Model file for the job. Use its own axes, mm. A direction names the side the tool comes from. Coordinates: 2 decimals unless noted, no trailing zeros. Write each loop counter-clockwise with the first axis right and the second up, starting at its lowest first coordinate (ties: lowest second). Pieces come first, ordered by that corner, then holes. Notation, with made-up numbers: M -3.75,54 L 49.25,54 A29 cw 49.25,74 Z; hole C 9.25,-6 d1. An arc over 180 degrees is marked long. Use CSV: the item, a comma, the result in double quotes. Start each with the question number.
Autodesk Fusion 360 part; units mm, degrees
sketch "Sketch1" plane through (0, 0, 0) normal (0, 0, 1) x (1, 0, 0)
  line L0 (0, 0) -> (20, 0)
  line L1 (20, 0) -> (20, 11)
  line L2 (20, 11) -> (0, 11)
  line L3 (0, 11) -> (0, 0)
  line L4 (0, 0) -> (80, 0)
  line L5 (0, 11) -> (0, 26)
  line L6 (0, 26) -> (80, 26)
  line L7 (80, 26) -> (80, 0)
  line L8 (80, 0) -> (0, 0)
  line L9 (0, 0) -> (0, 26)
  line L10 (80, 0) -> (80, -10)
  line L11 (80, -10) -> (0, -10)
  line L12 (0, -10) -> (0, 0)
  point P0 (5.75, 9.5)
  point P1 (14.25, 9.5)
  point P2 (14.25, 1.5)
  point P3 (5.75, 1.5)
  dimension "d1" = 20
  dimension "d2" = 11
  dimension "d3" = 1.5
  dimension "d4" = 1.5
  dimension "d5" = 8.5
  dimension "d6" = 5.75
  dimension "d7" = 80
  dimension "d8" = 15
  dimension "d19" = 10
extrude "Extrude1" add sketch "Sketch1" along normal blind 5
hole "Hole1" at (14.25, 1.5, 0) direction (0, 0, 1) diameter 2 end through all
pattern_linear "R-Pattern1" count 2 spacing 8.5 along (-1, 0, 0) count 2 spacing 8 along (0, 1, 0) of "Hole1"
sketch "Sketch2" plane through (0, 26, 0) normal (0, 1, 0) x (-1, 0, 0)
  line L0 (-80, 0) -> (0, 0)
  line L1 (0, 0) -> (0, 5)
  line L2 (0, 5) -> (-80, 5)
  line L3 (-80, 5) -> (-80, 0)
  circle A0 centre (-65, 25) radius 8
  line L4 (-73, 25) -> (-73, 5)
  line L5 (-57, 25) -> (-57, 5)
  line L6 (-57, 5) -> (-73, 5)
  circle A1 centre (-65, 25) radius 10
  line L7 (-75, 25) -> (-75, 5)
  line L8 (-55, 25) -> (-55, 5)
  dimension "d24" = 16
  dimension "d25" = 7
  dimension "d27" = 20
  dimension "d28" = 2
  dimension "d29" = 2
  dimension "d30" = -2
extrude "Extrude2" add sketch "Sketch2" against normal blind 5 contours L2 L4 A1 L7 | L2 L5 A1 L8 | L2 L4 L5 L6 A1 | A0 L4 L5 A1 | A0 L4 L5 A1
ref_plane "WorkPlane2" through (65, 15.5, 20) normal (0, -1, 0) x (1, 0, 0)
mirror "Mirror1" about plane through (65, 15.5, 20) normal (0, -1, 0) of "Extrude2"
equation "d33 = ( 11 / 2 ) * 1 mm"
1) Two-plate mould, pull along X, no slides. Class faces 1 (the face through (80, 8, 2)), 2 (the face through (39, 8, 5)), 3 (the face through (15.226, 1.283, 2.535)): pulls with the +X half, pulls with the -X half, needs draft (parallel to the pull), parting line crosses it, or undercut.
2) Band-saw the part on B-B on z = 12.5. List the corners of the cut face in (x, y).
3) Band-saw the part on D-D on z = 29.5. List the corners of the cut face in (x, y), then the cut area to 3 significant figures.
4) Band-saw the part on C-C on y = 1.5. List the corners of the cut face in (x, z), then the cut area to 3 significant figures.
5) Band-saw the part on A-A on x = 14.25. List the corners of the cut face in (y, z), then the cut area to 3 significant figures.
6) Wall check: L1, parallel to X at y = 9.5, z = 1.15; L2, parallel to Z at x = 65, y = 22.2; L3, parallel to Y at x = 14.25, z = 3.75. Give the ranges that are in metal, low to high. Write a range as [from, to].
7) Drop flat-ended pins along their axis: P1, Ø16, axis at x = 66.5, z = 23.5, coming from the +Y side; P2, Ø16, axis at x = 62, z = 25.5, coming from the -Y side; P3, Ø11, axis at x = 22, y = 14.5, coming from the +Z side; P4, Ø5.5, axis at y = 22.5, z = 17, coming from the +X side. Give the stop position or say it passes through.
8) Tool access for faces 4 (the face through (75, 7, 15)), 5 (the face through (67, 21, 17)), 6 (the face through (63, 5, 17)): list every direction of +Z, -Z, +X, -X, +Y, -Y with a clear straight run to the whole face (end or side of a thin tool).
Findings below:
1,face 1,"pulls with the +X half"
1,face 2,"needs draft"
1,face 3,"undercut"
2,outline,"M 55,5 L 75,5 L 75,10 L 55,10 Z; M 55,21 L 75,21 L 75,26 L 55,26 Z"
3,outline,"M 56.07,5 L 58.39,5 L 58.39,10 L 56.07,10 Z; M 56.07,21 L 58.39,21 L 58.39,26 L 56.07,26 Z; M 71.61,5 L 73.93,5 L 73.93,10 L 71.61,10 Z; M 71.61,21 L 73.93,21 L 73.93,26 L 71.61,26 Z"
3,area,"46.3 mm2"
4,outline,"M 0,0 L 4.75,0 L 4.75,5 L 0,5 Z; M 6.75,0 L 13.25,0 L 13.25,5 L 6.75,5 Z; M 15.25,0 L 80,0 L 80,5 L 15.25,5 Z"
4,area,"380 mm2"
5,outline,"M -10,0 L 0.5,0 L 0.5,5 L -10,5 Z; M 2.5,0 L 8.5,0 L 8.5,5 L 2.5,5 Z; M 10.5,0 L 26,0 L 26,5 L 10.5,5 Z"
5,area,"160 mm2"
6,L1,"x = [0, 4.75], [6.75, 13.25], [15.25, 80]"
6,L2,"z = [0, 17], [33, 35]"
6,L3,"y = [-10, 0.5], [2.5, 8.5], [10.5, 26]"
7,P1,"stops at y = 26"
7,P2,"stops at y = 5"
7,P3,"stops at z = 5"
7,P4,"stops at x = 75"
8,face 4,"+Z, +X, +Y, -Y"
8,face 5,"+Z, +X, -X"
8,face 6,"+Z, +X, -X, -Y"
